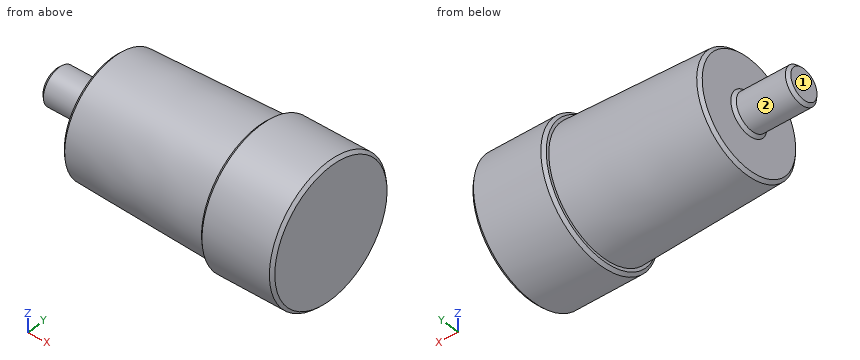
Autodesk Fusion 360 part; units mm, degrees
sketch "Sketch1" plane through (0, 0, 0) normal (0, 1, 0) x (1, 0, 0)
  line L0 (0, 0) -> (0, -10.033)
  line L1 (25.4, -10.92) -> (25.4, -11.938)
  line L2 (25.4, -11.938) -> (38.1, -11.938)
  line L3 (38.1, -11.938) -> (38.1, 0)
  line L4 (38.1, 0) -> (0, 0)
  line L5 (25.4, -10.92) -> (0, -10.033)
  line L6 (0, -3.175) -> (-9.525, -3.175)
  line L7 (-9.525, -3.175) -> (-9.525, 0)
  line L8 (-9.525, 0) -> (0, 0)
  dimension "d1" = 10.033
  dimension "d2" = 25.4
  dimension "d3" = 12.7
  dimension "d4" = 11.938
  dimension "d5" = 92
  dimension "d7" = 3.175
  dimension "d8" = 9.525
revolve "Revolve1" add sketch "Sketch1" angle 360 about axis through (38.1, 0, 0) along (-1, 0, 0)
chamfer "Chamfer1" distance 0.508 angle 45 5 edges at (-9.525, -1.1481, -2.9601) (0, -1.1481, -2.9601) (0, -3.6281, -9.354) (25.4, -4.317, -11.1301) (38.1, -4.317, -11.1301)
Read the model definition and answer for the solid it produces. Units are mm, in the model's axes. Face numbers are marked on the shaded views. A direction names the side the tool comes from. Coordinates: 2 decimals unless noted, no trailing zeros. Loops run counter-clockwise (first coordinate to the right, second up) from the corner with the lowest first, then second, coordinate; pieces in that order, holes last. Notation, with made-up numbers: (66.5, 81.5) - (78.5, 81.5) arc R18 cw to (78.5, 96.5) - close; hole circle Ø9 at (27, 40.5). An arc over 180 degrees is marked (long way). Answer in a Markdown table with one row per item.
1. Find section B-B, the plane x = 1. Write down the section's boundary in (y, z), then the cut area to 3 significant figures.
Conclusion:
| item | result |
|---|---|
| outline | circle Ø20.14 at (0, 0) |
| area | 318 mm² |
2. Find section A-A, the plane z = 0. Write down the section's boundary in (x, y) (3 decimals).
Conclusion:
| item | result |
|---|---|
| outline | (-9.525, -2.667) - (-9.017, -3.175) - (-0.508, -3.175) - (0, -3.683) - (0, -9.525) - (0.508, -10.051) - (25.4, -10.92) - (25.4, -11.43) - (25.908, -11.938) - (37.592, -11.938) - (38.1, -11.43) - (38.1, 11.43) - (37.592, 11.938) - (25.908, 11.938) - (25.4, 11.43) - (25.4, 10.92) - (0.508, 10.051) - (0, 9.525) - (0, 3.683) - (-0.508, 3.175) - (-9.017, 3.175) - (-9.525, 2.667) - close |
3. Which of the six approach directions +Z, -Z, +X, -X, +Y, -Y give full straight-line access (tool end or side, diameter ignored) to the marked faces 1 and 2?
Conclusion:
| item | result |
|---|---|
| face 1 | +Z, -Z, -X, +Y, -Y |
| face 2 | -X |
4. Straight lines are drawn through the part: line 1 (X direction, y = 4.5, z = -1.25); line 2 (Y direction, x = 25, z = -1); line 3 (Z direction, x = 33, y = 1.5). For each, find the intervals that lie inside material, in ascending order.
Conclusion:
| item | result |
|---|---|
| line 1 | x = 0 to 38.1 |
| line 2 | y = -10.86 to 10.86 |
| line 3 | z = -11.84 to 11.84 |
5. Given pin 1 (2 mm diameter, centred on x = 22.5, y = 2.5, fed in from +Z); pin 2 (5 mm diameter, centred on x = 16, y = 2.5, fed in from -Z); pin 3 (2 mm diameter, centred on x = 32.5, y = 7, fed in from +Z), each flat-ended and moving along its own axis, determine where each tip first touches the part or whether it passes through.
Conclusion:
| item | result |
|---|---|
| pin 1 | stops at z = 10.72 |
| pin 2 | stops at z = -10.63 |
| pin 3 | stops at z = 10.32 |
6. Find section C-C, the plane x = 18.5. Write down the section's boundary in (y, z).
Conclusion:
| item | result |
|---|---|
| outline | circle Ø21.36 at (0, 0) |
